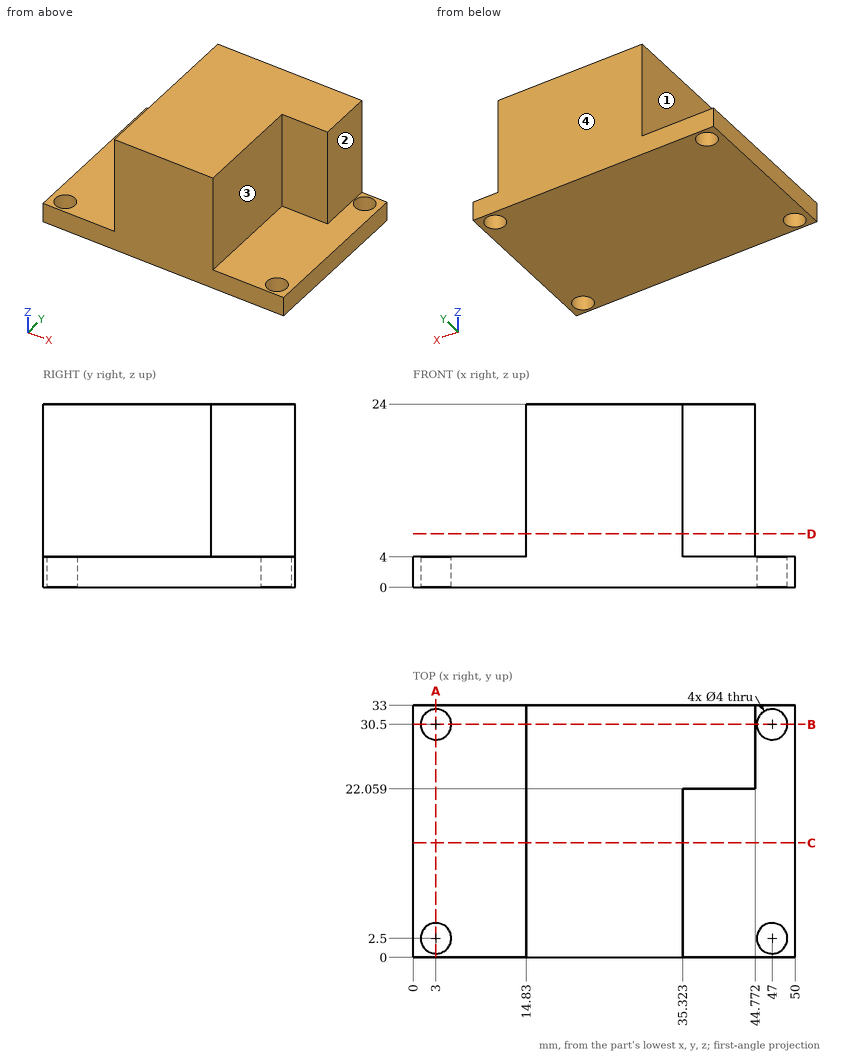
For this review, use the dimensioned drawing (mm, ordinates from the lowest corner) and the shaded views. A direction names the side the tool comes from. Give positions to 0.01 mm unless a question says otherwise; leave off trailing zeros. Order: outer loops, then holes, each group sorted by start corner. A loop starts at its lowest first (then second) coordinate and runs counter-clockwise, first axis right, second up.
1) For the marked faces 1, 2, 3 and 4, list the 3-axis set-ups (+Z, -Z, +X, -X, +Y, -Y) from which the entire face can be reached by the end or side of a thin tool; tool diameter is ignored.
2) Take a section at C-C (y = 15). Give the boundary of the cut face in (x, z), then the cut area to 3 significant figures.
3) Take a section at D-D (z = 7). Give the boundary of the cut face in (x, y).
4) Wall thickness on line 1 (Y direction, x = 47, z = 2.15); line 2 (Z direction, x = 5.5, y = 19); line 3 (X direction, y = 19, z = 18.25): over which ranges is each line inside the solid? List them lowest first.
5) Insertion check: pin 1 (2 mm diameter, centred on x = 10, z = 3, fed in from -Y); pin 2 (3.5 mm diameter, centred on x = 3, y = 30.5, fed in from -Z); pin 3 (5 mm diameter, centred on x = 47, y = 2.5, fed in from +Z); pin 4 (1.5 mm diameter, centred on y = 9.5, z = 14.5, fed in from +X). Each pin has a flat end and moves straight along its axis. Give the tip position at first contact, or say it passes through.
6) Take a section at B-B (y = 30.5). Give the boundary of the cut face in (x, z), then the cut area to 3 significant figures.
7) Take a section at A-A (x = 3). Give the boundary of the cut face in (y, z).
Derived:
1. face 1: +Z, -X, +Y, -Y
1. face 2: +Z, +X, +Y, -Y
1. face 3: +Z, +X, -Y
1. face 4: +Z, -Z, +X, -X, +Y
2. outline: (0, 0) - (50, 0) - (50, 4) - (35.32, 4) - (35.32, 24) - (14.83, 24) - (14.83, 4) - (0, 4) - close
2. area: 610 mm2
3. outline: (14.83, 0) - (35.32, 0) - (35.32, 22.06) - (44.77, 22.06) - (44.77, 33) - (14.83, 33) - close
4. line 1: y = 0 to 0.5, 4.5 to 28.5, 32.5 to 33
4. line 2: z = 0 to 4
4. line 3: x = 14.83 to 35.32
5. pin 1: stops at y = 0
5. pin 2: passes through
5. pin 3: stops at z = 4
5. pin 4: stops at x = 35.32
6. outline: (0, 0) - (1, 0) - (1, 4) - (0, 4) - close; (5, 0) - (45, 0) - (45, 4) - (44.77, 4) - (44.77, 24) - (14.83, 24) - (14.83, 4) - (5, 4) - close; (49, 0) - (50, 0) - (50, 4) - (49, 4) - close
6. area: 767 mm2
7. outline: (0, 0) - (0.5, 0) - (0.5, 4) - (0, 4) - close; (4.5, 0) - (28.5, 0) - (28.5, 4) - (4.5, 4) - close; (32.5, 0) - (33, 0) - (33, 4) - (32.5, 4) - close
